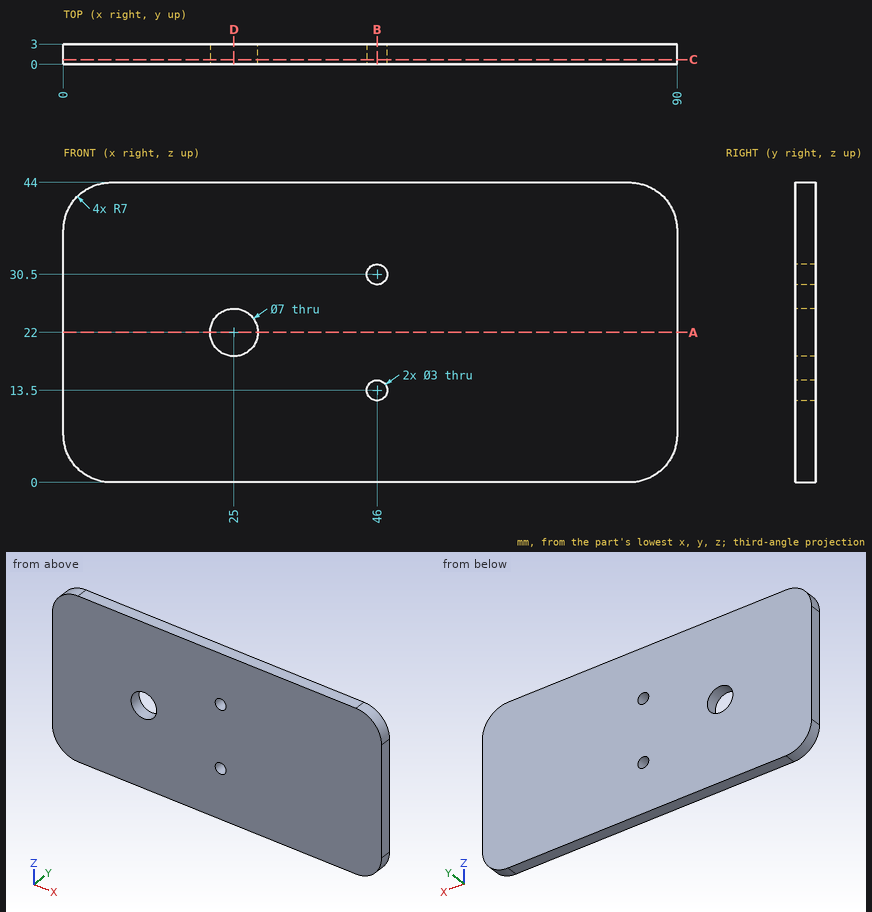
Part print with two shaded views. Sizes in mm from the minimum x, y, z corner. Round coordinates to 2 decimals unless told otherwise and drop trailing zeros. Write each loop counter-clockwise with the first axis right and the second up, starting at its lowest first coordinate (ties: lowest second). Pieces come first, ordered by that corner, then holes. Notation, with made-up numbers: (-16.5, -28) - (37.5, -28) arc R30 ccw to (37.5, -1) - close; hole circle Ø4 at (89, 17). An arc over 180 degrees is marked (long way). Answer as CSV lines item,"result".
Q1. Drop a flat-ended pin along its axis: pin 1 (1.5 mm diameter, centred on y = 1, z = 6.5, fed in from +X). Give the stop position or say it passes through.
Report:
pin 1,"stops at x = 90"
Q2. Cut at A-A (z = 22). Write the cut outline in (x, y), and give its area (3 significant figures).
Report:
outline,"(0, 0) - (21.5, 0) - (21.5, 3) - (0, 3) - close; (28.5, 0) - (90, 0) - (90, 3) - (28.5, 3) - close"
area,"249 mm^2"
Q3. Cut at B-B (x = 46). Write the cut outline in (y, z).
Report:
outline,"(0, 0) - (3, 0) - (3, 12) - (0, 12) - close; (0, 15) - (3, 15) - (3, 29) - (0, 29) - close; (0, 32) - (3, 32) - (3, 44) - (0, 44) - close"
Q4. Drill centre lines: probe 1 along Z at (x, y) = (46, 1.9); probe 2 along Z at (x, y) = (25, 1.6); probe 3 along X at (y, z) = (1.9, 22). Where is each one in solid material? Low to high. Write a range as [from, to].
Report:
probe 1,"z = [0, 12], [15, 29], [32, 44]"
probe 2,"z = [0, 18.5], [25.5, 44]"
probe 3,"x = [0, 21.5], [28.5, 90]"
Q5. Cut at C-C (y = 0.7). Write the cut outline in (x, z), and give its area (3 significant figures).
Report:
outline,"(0, 7) arc R7 ccw to (7, 0) - (83, 0) arc R7 ccw to (90, 7) - (90, 37) arc R7 ccw to (83, 44) - (7, 44) arc R7 ccw to (0, 37) - close; hole circle Ø7 at (25, 22); hole circle Ø3 at (46, 13.5); hole circle Ø3 at (46, 30.5)"
area,"3,870 mm^2"
Q6. Cut at D-D (x = 25). Write the cut outline in (y, z).
Report:
outline,"(0, 0) - (3, 0) - (3, 18.5) - (0, 18.5) - close; (0, 25.5) - (3, 25.5) - (3, 44) - (0, 44) - close"
